Read the model definition and answer for the solid it produces. Units are mm, in the model's axes. A direction names the side the tool comes from. Give positions to 0.01 mm unless a question says otherwise; leave off trailing zeros. Loops run counter-clockwise (first coordinate to the right, second up) from the corner with the lowest first, then second, coordinate; pieces in that order, holes last.
(1) Find section A-A, the plane z = -16.5. Write down the section's boundary in (x, y), then the cut area to 3 significant figures.
(2) Each of these flat-tipped pins is pushed along its axis until it touches: P1, Ø1.5, axis at y = 51, z = -13, coming from the -X side; P2, Ø1, axis at x = 38, y = -1.5, coming from the +Z side; P3, Ø1, axis at x = 37, y = -1, coming from the -Z side; P4, Ø3, axis at x = 59, z = -13, coming from the -Y side (3 decimals). Where does it stop, or does it pass through?
(3) Determine the mould class of faces 1 (the face through (25.353, 66.07, -38.258)), 2 (the face through (45, -1, 2)) for opening direction Z: pulls with the +Z half, pulls with the -Z half, needs draft (parallel to the pull), parting line crosses it, or undercut.
(4) Find section D-D, the plane x = 18. Write down the section's boundary in (y, z), then the cut area to 3 significant figures.
(5) Which of the six approach directions +Z, -Z, +X, -X, +Y, -Y give full straight-line access (tool end or side, diameter ignored) to faces 3 (the face through (63.407, 67.056, -36.707)), 4 (the face through (45, 35, 4.2)), 5 (the face through (67.677, -1.014, -13.064))?
(6) Find section B-B, the plane y = 32.5. Write down the section's boundary in (x, z).
(7) Find section C-C, the plane x = 36. Write down the section's boundary in (y, z), then the cut area to 3 significant figures.
(8) Straight lines are drawn through the part: probe 1 along X at (y, z) = (13, -16); probe 2 along Y at (x, z) = (57, -52); probe 3 along X at (y, z) = (11, -58.5). For each, find the intervals that lie inside material, in ascending order.
```python
from build123d import *

# Parameters (mm, degrees)
BOSS_EXTRUDE1_DEPTH   = 71
BOSS_EXTRUDE1_2_DEPTH = 71
CUT_EXTRUDE1_START    = -71
CUT_EXTRUDE1_DEPTH    = 71
FILLET1_DEPTH         = 71
FILLET2_R             = 17.5
BOSS_EXTRUDE2_DEPTH   = 2
CUT_EXTRUDE2_REACH    = 128.609
SKETCH5_R             = 1.2
CUT_EXTRUDE3_DEPTH    = 10
CUT_EXTRUDE4_DEPTH    = 8
BOSS_EXTRUDE3_DEPTH   = 71
FILLET3_R             = 0.4
FILLET4_R             = 0.2


with BuildPart() as part:
    # Sketch1 → Boss-Extrude1 (new body)
    with BuildSketch(Plane(origin=(0, 0, 0), x_dir=(1, 0, 0), z_dir=(0, 1, 0))):
        Polygon((-3.464101615, -2), (93.621778265, -2), (45.078838325, 82.078838325), align=None)
        with BuildLine():
            ThreePointArc((53.328838206, 30.789419094), (75.868257522, 8.250000059), (45.078838325, 16.5))
            ThreePointArc((45.078838325, 16.5), (14.289419055, 8.250000187), (36.828838698, 30.789418947))
            ThreePointArc((36.828838698, 30.789418947), (45.078838178, 61.578838325), (53.328838206, 30.789419094))
        make_face(mode=Mode.SUBTRACT)
    extrude(amount=BOSS_EXTRUDE1_DEPTH)

    # Fillet1: read off the stored shape, not the designer's step
    # Fillet1 outline → Fillet1 (cut)
    with BuildSketch(Plane(origin=(0, 0, 0), x_dir=(1, 0, 0), z_dir=(0, 1, 0))):
        with BuildLine():
            ThreePointArc((53.328838325, 30.789419162), (60.354714381, 32.954528877), (67.623619549, 31.852870088))
            ThreePointArc((67.623619549, 31.852870088), (62.626869283, 36.157639839), (61.397204455, 42.637337381))
            ThreePointArc((61.397204455, 42.637337381), (58.716816368, 35.791451453), (53.328838325, 30.789419162))
        make_face()
        with BuildLine():
            ThreePointArc((38.852423231, 3.588630855), (45.078838325, 5.763558647), (51.305253419, 3.588630855))
            ThreePointArc((51.305253419, 3.588630855), (46.716736338, 9.332857994), (45.078838325, 16.5))
            ThreePointArc((45.078838325, 16.5), (43.440940312, 9.332857994), (38.852423231, 3.588630855))
        make_face()
        with BuildLine():
            ThreePointArc((36.828838325, 30.789419162), (31.440860282, 35.791451453), (28.760472195, 42.637337381))
            ThreePointArc((28.760472195, 42.637337381), (27.530807367, 36.157639839), (22.534057101, 31.852870089))
            ThreePointArc((22.534057101, 31.852870089), (29.802962269, 32.954528877), (36.828838325, 30.789419162))
        make_face()
    extrude(amount=FILLET1_DEPTH, mode=Mode.SUBTRACT)

    # Fillet2
    fillet2_edges = [part.edges().sort_by_distance(p)[0] for p in [
        (93.621778265, 35.5, 2),
        (-3.464101615, 35.5, 2),
        (45.078838325, 35.5, -82.078838325),
    ]]
    fillet(fillet2_edges, radius=FILLET2_R)

    # Sketch3 → Boss-Extrude2 (add)
    with BuildSketch(Plane.XZ):
        with BuildLine():
            Line((60.234282891, -55.828838325), (78.466333699, -24.25))
            ThreePointArc((78.466333699, -24.25), (78.466333699, -6.75), (63.310889132, 2))
            Line((63.310889132, 2), (26.846787517, 2))
            ThreePointArc((26.846787517, 2), (11.691342951, -6.75), (11.691342951, -24.25))
            Line((11.691342951, -24.25), (29.923393759, -55.828838325))
            ThreePointArc((29.923393759, -55.828838325), (45.078838325, -64.578838325), (60.234282891, -55.828838325))
        make_face()
    extrude(amount=BOSS_EXTRUDE2_DEPTH)

    # Sketch4 → Cut-Extrude2 (cut, up to next)
    with BuildSketch(Plane.XZ.offset(2), mode=Mode.PRIVATE) as cut_extrude2_sk1:
        with BuildLine():
            Line((63.310889132, -10.5), (26.846787517, -10.5))
            ThreePointArc((26.846787517, -10.5), (22.516660498, -13), (22.516660498, -18))
            Line((22.516660498, -18), (40.748711306, -49.578838325))
            ThreePointArc((40.748711306, -49.578838325), (45.078838325, -52.078838325), (49.408965344, -49.578838325))
            Line((49.408965344, -49.578838325), (67.641016151, -18))
            ThreePointArc((67.641016151, -18), (67.641016151, -13), (63.310889132, -10.5))
        make_face()
    cut_extrude2_tool1 = extrude(cut_extrude2_sk1.sketch, amount=-CUT_EXTRUDE2_REACH, mode=Mode.PRIVATE) & part.part
    add(cut_extrude2_tool1.solids().sort_by_distance((45.078838, -2, -26.026279))[0], mode=Mode.SUBTRACT)

    # Sketch5 → Cut-Extrude3 (cut)
    with BuildSketch(Plane(origin=(0, 71, 0), x_dir=(1, 0, 0), z_dir=(0, 1, 0))):
        with Locations(Location((45.078838325, 1.875, 0), (0, 0, 270))):
            Circle(SKETCH5_R)
        with Locations(Location((24.163216795, 38.101919162, 0), (0, 0, 270))):
            Circle(SKETCH5_R)
        with Locations(Location((65.994459855, 38.101919162, 0), (0, 0, 270))):
            Circle(SKETCH5_R)
    extrude(amount=-CUT_EXTRUDE3_DEPTH, mode=Mode.SUBTRACT)

    # Sketch7 → Cut-Extrude4 (cut)
    with BuildSketch(Plane(origin=(0, 71, 0), x_dir=(1, 0, 0), z_dir=(0, 1, 0))):
        with BuildLine():
            ThreePointArc((50.713743985, 2.845248996), (45.078838325, 4.813558647), (39.443932665, 2.845248996))
            ThreePointArc((39.443932665, 2.845248996), (13.466695029, 7.775), (22.186024243, 32.736823215))
            ThreePointArc((22.186024243, 32.736823215), (26.708083233, 36.632639839), (27.820929903, 42.496766114))
            ThreePointArc((27.820929903, 42.496766114), (45.078838325, 62.528838325), (62.336746747, 42.496766114))
            ThreePointArc((62.336746747, 42.496766114), (63.449593417, 36.632639839), (67.971652407, 32.736823215))
            ThreePointArc((67.971652407, 32.736823215), (76.690981621, 7.775), (50.713743985, 2.845248996))
        make_face()
    extrude(amount=-CUT_EXTRUDE4_DEPTH, mode=Mode.SUBTRACT)

    # Sketch8 → Boss-Extrude3 (add, through all)
    with BuildSketch(Plane(origin=(0, 0, 0), x_dir=(1, 0, 0), z_dir=(0, 1, 0))):
        Polygon((63.310889132, -2), (63.310889132, -3), (64.110889132, -3.8), (64.110889132, -4.2), (26.046787517, -4.2), (26.046787517, -3.8), (26.846787517, -3), (26.846787517, -2), align=None)
    extrude(amount=BOSS_EXTRUDE3_DEPTH)

    # Fillet3
    fillet3_edges = [part.edges().sort_by_distance(p)[0] for p in [
        (63.310889132, 35.5, 2),
        (26.846787517, 35.5, 3),
        (63.310889132, 35.5, 3),
        (26.846787517, 35.5, 2),
    ]]
    fillet(fillet3_edges, radius=FILLET3_R)

    # Fillet4
    fillet4_edges = [part.edges().sort_by_distance(p)[0] for p in [
        (26.046787517, 35.5, 3.8),
        (26.046787517, 35.5, 4.2),
        (64.110889132, 35.5, 4.2),
        (64.110889132, 35.5, 3.8),
    ]]
    fillet(fillet4_edges, radius=FILLET4_R)


with BuildPart() as body_2:
    # Sketch1 → Boss-Extrude1 2 (new body)
    with BuildSketch(Plane(origin=(0, 0, 0), x_dir=(1, 0, 0), z_dir=(0, 1, 0))):
        with BuildLine():
            ThreePointArc((36.828838698, 30.789418947), (42.868257595, 24.749999813), (45.078838325, 16.5))
            ThreePointArc((45.078838325, 16.5), (47.289419128, 24.749999941), (53.328838206, 30.789419094))
            ThreePointArc((53.328838206, 30.789419094), (45.078838472, 28.578838325), (36.828838698, 30.789418947))
        make_face()
    extrude(amount=BOSS_EXTRUDE1_2_DEPTH)

    # Sketch2 → Cut-Extrude1 (cut)
    with BuildSketch(Plane(origin=(0, 71, 0), x_dir=(1, 0, 0), z_dir=(0, 1, 0)).offset(CUT_EXTRUDE1_START)):
        with BuildLine():
            ThreePointArc((36.828838325, 30.789419162), (45.078838325, 28.578838325), (53.328838325, 30.789419162))
            ThreePointArc((53.328838325, 30.789419162), (47.289419162, 24.75), (45.078838325, 16.5))
            ThreePointArc((45.078838325, 16.5), (42.868257487, 24.75), (36.828838325, 30.789419162))
        make_face()
    extrude(amount=CUT_EXTRUDE1_DEPTH, mode=Mode.SUBTRACT)


solid = part.part
```
Entries:
1. outline: (9.38, -2) - (21.95, -2) - (21.95, 0) - (12.08, 0) - (12.08, 63) - (11.13, 63) - (11.13, 71) - (9.38, 71) - close; (68.21, -2) - (80.78, -2) - (80.78, 71) - (79.03, 71) - (79.03, 63) - (78.08, 63) - (78.08, 0) - (68.21, 0) - close
1. area: 419 mm2
2. P1: stops at x = 9.43
2. P2: stops at z = 2
2. P3: stops at z = -62.85
2. P4: passes through
3. face 1: undercut
3. face 2: pulls with the +Z half
4. outline: (-2, -35.18) - (71, -35.18) - (71, -30.38) - (63, -30.38) - (63, -29.16) - (0, -29.16) - (0, -3.84) - (63, -3.84) - (63, -2.62) - (71, -2.62) - (71, -0.4) - (-2, -0.4) - close
4. area: 721 mm2
5. face 3: +Y
5. face 4: +Z, +X, -X, +Y, -Y
5. face 5: +Y, -Y
6. outline: (11.69, -24.25) - (29.92, -55.83) arc R17.5 ccw to (60.23, -55.83) - (78.47, -24.25) arc R17.5 ccw to (63.7, 2) arc R0.4 cw to (63.31, 2.4) - (63.31, 2.83) arc R0.4 cw to (63.43, 3.12) - (64.05, 3.74) arc R0.2 ccw to (64.11, 3.88) - (64.11, 4) arc R0.2 ccw to (63.91, 4.2) - (26.25, 4.2) arc R0.2 ccw to (26.05, 4) - (26.05, 3.88) arc R0.2 ccw to (26.11, 3.74) - (26.73, 3.12) arc R0.4 cw to (26.85, 2.83) - (26.85, 2.4) arc R0.4 cw to (26.46, 2) arc R17.5 ccw to start; hole (22.53, -31.85) arc R10 cw to (28.76, -42.64) arc R16.5 ccw (long way) to (61.4, -42.64) arc R10 cw to (67.62, -31.85) arc R16.5 ccw (long way) to (51.31, -3.59) arc R10 cw to (38.85, -3.59) arc R16.5 ccw (long way) to start
7. outline: (-2, -62.04) - (71, -62.04) - (71, -59.98) - (63, -59.98) - (63, -58.86) - (0, -58.86) - (0, -41.35) - (-2, -41.35) - close; (-2, -10.5) - (0, -10.5) - (0, -1.76) - (63, -1.76) - (63, -0.71) - (71, -0.71) - (71, 4.2) - (0, 4.2) - (0, 2) - (-2, 2) - close
7. area: 698 mm2
8. probe 1: x = 9.35 to 12.09, 78.07 to 80.8
8. probe 2: y = -2 to 0
8. probe 3: x = 31.82 to 35.48, 54.68 to 58.34
